Autodesk Inventor part; units mm, degrees
ref_plane "Work Plane1" through (-457.2, 0, 457.2) normal (1, 0, 0) x (0, 1, 0)
ref_plane "YZ Plane" through (0, 0, 0) normal (1, 0, 0) x (0, 1, 0)
ref_plane "XZ Plane" through (0, 0, 0) normal (0, 1, 0) x (-1, 0, 0)
sketch "Sketch1" plane through (0, 0, 0) normal (0, 1, 0) x (-1, 0, 0)
  line L0 (0, 0) -> (914.4, 0)
  line L1 (914.4, 0) -> (914.4, 25.4)
  line L2 (914.4, 25.4) -> (889, 25.4)
  line L3 (889, 25.4) -> (914.4, 0)
  line L4 (889, 25.4) -> (25.4, 25.4)
  line L5 (25.4, 25.4) -> (0, 0)
  dimension "d0" = 914.4
  dimension "d1" = 25.4
  dimension "d2" = 25.4
  dimension "d3" = 863.6
extrude "Extrusion1" add sketch "Sketch1" along normal blind 50.8 contours L5 L4 L3 L0
ref_plane "Work Plane1" through (-457.2, 0, 457.2) normal (1, 0, 0) x (0, 1, 0)
sketch "Sketch2" plane through (-457.2, 0, 457.2) normal (1, 0, 0) x (0, 1, 0)
  line L0 (50.8, -457.2) -> (47.625, -457.2)
  line L1 (0, -457.2) -> (50.8, -457.2)
  line L2 (47.625, -457.2) -> (47.625, -454.025)
  line L3 (47.625, -454.025) -> (3.175, -454.025)
  line L4 (3.175, -454.025) -> (3.175, -434.975)
  line L5 (3.175, -434.975) -> (47.625, -434.975)
  line L6 (47.625, -434.975) -> (47.625, -454.025)
  dimension "d6" = 3.175
  dimension "d7" = 3.175
  dimension "d8" = 44.45
  dimension "d9" = 19.05
extrude "Extrusion2" cut sketch "Sketch2" along normal through all both and the other way through all
properties part number "36in 2x1 double corner"
Check sheet for the modelled part. Datum: model origin and axes. Units: mm. A direction names the side the tool comes from. Coordinates: 2 decimals unless noted, no trailing zeros. Write each loop counter-clockwise with the first axis right and the second up, starting at its lowest first coordinate (ties: lowest second). Pieces come first, ordered by that corner, then holes. Notation, with made-up numbers: (6.25, 55.25) - (17.25, 55.25) arc R10 cw to (17.25, 66.25) - close; hole circle Ø8 at (39, -16). An arc over 180 degrees is marked (long way). One line per question, with ' | ' between items.
Item 1: Sectioned sample at C-C on x = -369. Record the boundary of the cut face in (y, z) (3 decimals), plus the area to 3 significant figures.
Determined:
outline: (0, 0) - (50.8, 0) - (50.8, 25.4) - (0, 25.4) - close; hole (3.175, 3.175) - (47.625, 3.175) - (47.625, 22.225) - (3.175, 22.225) - close | area: 444 mm2
Item 2: Mould release check, pull along Y, two halves, no side actions. Record for faces 3 (the face through (-451, 0, 13)), 4 (the face through (-463, 25, 22.225)), 5 (the face through (-463, 25, 25.4)), 6 (the face through (-451, 50.8, 13)): pulls with the +Y half, pulls with the -Y half, needs draft (parallel to the pull), parting line crosses it, or undercut.
Determined:
face 3: pulls with the -Y half | face 4: undercut | face 5: needs draft | face 6: pulls with the +Y half
Item 3: Sectioned sample at A-A on z = 12.5. Record the boundary of the cut face in (x, y) (3 decimals).
Determined:
outline: (-901.9, 0) - (-12.5, 0) - (-12.5, 3.175) - (-901.9, 3.175) - close; (-901.9, 47.625) - (-12.5, 47.625) - (-12.5, 50.8) - (-901.9, 50.8) - close
Item 4: Thickness scan on line 1 (Y direction, x = -113.5, z = 4) (3 decimals); line 2 (Z direction, x = -868.5, y = 19) (3 decimals); line 3 (X direction, y = 48.5, z = 20.75). Record the ranges inside material, lowest first. Write a range as [from, to].
Determined:
line 1: y = [0, 3.175], [47.625, 50.8] | line 2: z = [0, 3.175], [22.225, 25.4] | line 3: x = [-893.65, -20.75]
Item 5: Gauge pin test, flat ends, axial feed: P1, Ø12, axis at y = 44.5, z = 20.5, coming from the -X side; P2, Ø12, axis at y = 12.5, z = 15.5, coming from the +X side. Record the tip position at first contact, or that the pin passes through.
Determined:
P1: stops at x = -899.02 | P2: passes through
Item 6: Access from +Z, -Z, +X, -X, +Y, -Y to the whole of each face (thin tool, end or side, straight path). Record for faces 1 (the face through (-23, 27, 23)), 2 (the face through (-464, 3.175, 13)).
Determined:
face 1: +Z, +X, +Y, -Y | face 2: +X, -X
Item 7: Sectioned sample at B-B on y = 40. Record the boundary of the cut face in (x, z) (3 decimals).
Determined:
outline: (-914.4, 0) - (0, 0) - (-3.175, 3.175) - (-911.225, 3.175) - close; (-892.175, 22.225) - (-22.225, 22.225) - (-25.4, 25.4) - (-889, 25.4) - close
